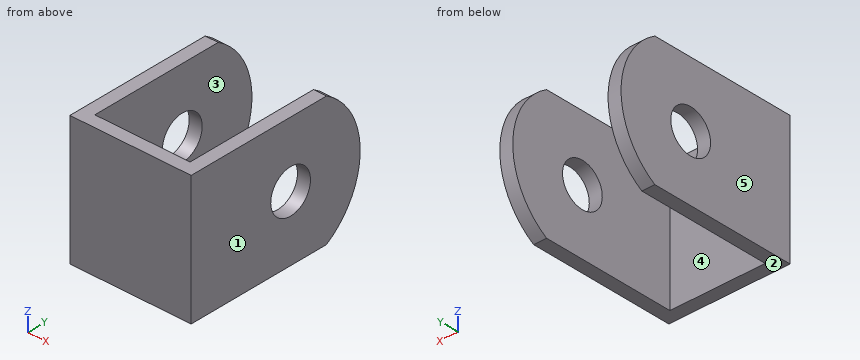
from build123d import *

# Parameters (mm, degrees)
SKETCH1_W           = 22
SKETCH1_H           = 35
BOSS_EXTRUDE1_DEPTH = 3
SKETCH2_W           = 35
SKETCH2_H           = 3
BOSS_EXTRUDE6_DEPTH = 3
BOSS_EXTRUDE7_START = 3
SKETCH4_W           = 35
SKETCH4_H           = 3
BOSS_EXTRUDE7_DEPTH = 3
SKETCH5_W           = 28
SKETCH5_H           = 2.5
CUT_EXTRUDE1_DEPTH  = 50


with BuildPart() as part:
    # Sketch1 → Boss-Extrude1 (new body)
    with BuildSketch(Plane(origin=(0, 0, 0), x_dir=(1, 0, 0), z_dir=(0, 1, 0))):
        with Locations((-45.186046512, -0.081395349)):
            Rectangle(SKETCH1_W, SKETCH1_H)
    extrude(amount=BOSS_EXTRUDE1_DEPTH)

    # Sketch2 → Boss-Extrude6 (add)
    with BuildSketch(Plane(origin=(-34.186046512, 0, 0), x_dir=(0, 0, -1), z_dir=(1, 0, 0))):
        with BuildLine():
            ThreePointArc((17.418604651, 25), (-0.081395349, 42.5), (-17.581395349, 25))
            Line((-17.581395349, 25), (-5.081395349, 25))
            ThreePointArc((-5.081395349, 25), (-0.081395349, 30), (4.918604651, 25))
            Line((4.918604651, 25), (17.418604651, 25))
        make_face()
        with BuildLine():
            Line((-5.081395349, 25), (-17.581395349, 25))
            ThreePointArc((-17.581395349, 25), (-0.081395349, 7.5), (17.418604651, 25))
            Line((17.418604651, 25), (4.918604651, 25))
            ThreePointArc((4.918604651, 25), (-0.081395349, 20), (-5.081395349, 25))
        make_face()
        with BuildLine():
            Line((-17.581395349, 25), (-17.581395349, 3))
            Line((-17.581395349, 3), (17.418604651, 3))
            Line((17.418604651, 3), (17.418604651, 25))
            ThreePointArc((17.418604651, 25), (-0.081395349, 7.5), (-17.581395349, 25))
        make_face()
        with Locations((-0.081395349, 1.5)):
            Rectangle(SKETCH2_W, SKETCH2_H)
    extrude(amount=BOSS_EXTRUDE6_DEPTH)

    # Sketch4 → Boss-Extrude7 (add)
    with BuildSketch(Plane.ZY.offset(56.186046512).offset(BOSS_EXTRUDE7_START)):
        with BuildLine():
            ThreePointArc((17.581395349, 25), (0.081395349, 42.5), (-17.418604651, 25))
            Line((-17.418604651, 25), (-4.918604651, 25))
            ThreePointArc((-4.918604651, 25), (0.081395349, 30), (5.081395349, 25))
            Line((5.081395349, 25), (17.581395349, 25))
        make_face()
        with BuildLine():
            Line((-4.918604651, 25), (-17.418604651, 25))
            ThreePointArc((-17.418604651, 25), (0.081395349, 7.5), (17.581395349, 25))
            Line((17.581395349, 25), (5.081395349, 25))
            ThreePointArc((5.081395349, 25), (0.081395349, 20), (-4.918604651, 25))
        make_face()
        with BuildLine():
            Line((-17.418604651, 25), (-17.418604651, 3))
            Line((-17.418604651, 3), (17.581395349, 3))
            Line((17.581395349, 3), (17.581395349, 25))
            ThreePointArc((17.581395349, 25), (0.081395349, 7.5), (-17.418604651, 25))
        make_face()
        with Locations((0.081395349, 1.5)):
            Rectangle(SKETCH4_W, SKETCH4_H)
    extrude(amount=-BOSS_EXTRUDE7_DEPTH)

    # Sketch5 → Cut-Extrude1 (cut)
    with BuildSketch(Plane.XZ):
        with Locations((-45.186046512, 16.331395349)):
            Rectangle(SKETCH5_W, SKETCH5_H)
        with Locations((-45.186046512, -16.168604651)):
            Rectangle(SKETCH5_W, SKETCH5_H)
    extrude(amount=-CUT_EXTRUDE1_DEPTH, mode=Mode.SUBTRACT)


solid = part.part
The model under review builds one solid part; all positions refer to its coordinate system, in mm. Face numbers are marked on the shaded views. A direction names the side the tool comes from. Round coordinates to 2 decimals unless told otherwise and drop trailing zeros. Write each loop counter-clockwise with the first axis right and the second up, starting at its lowest first coordinate (ties: lowest second). Pieces come first, ordered by that corner, then holes. Notation, with made-up numbers: M 26.25,79.25 L 58.25,79.25 A32 cw 58.25,109.25 Z; hole C 66,-6 d6. An arc over 180 degrees is marked long. Use a Markdown table: item, result. Add a question column.
Q1. We need section C-C, the plane z = 1.5. State the section outline as (x, y) points, plus the area to 3 significant figures.
Q2. To check wall thickness, follow line 1 (Z direction, x = -58, y = 25); line 2 (X direction, y = 34, z = -5); line 3 (Y direction, x = -36.75, z = -6). State the ranges of each line that lie inside material, in increasing order.
Q3. We need section D-D, the plane x = -33.5. State the section outline as (y, z) points, plus the area to 3 significant figures.
Q4. We need section A-A, the plane y = 25. State the section outline as (x, z) points.
Q5. We need section B-B, the plane y = 4.5. State the section outline as (x, z) points, plus the area to 3 significant figures.
Q6. The part is to be moulded in two halves that separate along X. For the marked faces 1, 2 and 3, say which applies: pulls with the +X half, pulls with the -X half, needs draft (parallel to the pull), parting line crosses it, or undercut.
Q7. Machinability: for the marked faces 4 and 5, which of the approach directions +Z, -Z, +X, -X, +Y, -Y give a long, thin tool a straight path to every point of the face, cutting with its end or side? Answer none if there is none.
Q8. Insertion check: pin 1 (8 mm diameter, centred on y = 25, z = 0.08, fed in from -X); pin 2 (11 mm diameter, centred on x = -48.5, z = -5.5, fed in from +Y). Each pin has a flat end and moves straight along its axis. Give the tip position at first contact, or say it passes through.
Findings below:
| question | item | result |
|---|---|---|
| 1 | outline | M -59.19,0 L -31.19,0 L -31.19,20.21 L -34.19,20.21 L -34.19,3 L -56.19,3 L -56.19,20.21 L -59.19,20.21 Z; M -59.19,29.79 L -56.19,29.79 L -56.19,42.44 L -59.19,42.44 Z; M -34.19,29.79 L -31.19,29.79 L -31.19,42.44 L -34.19,42.44 Z |
| 1 | area | 263 mm² |
| 2 | line 1 | z = -14.92 to -4.92, 5.08 to 15.08 |
| 2 | line 2 | x = -59.19 to -56.19, -34.19 to -31.19 |
| 2 | line 3 | y = 0 to 3 |
| 3 | outline | M 0,-14.92 L 34.01,-14.92 A17.5 ccw 34.01,15.08 L 0,15.08 Z; hole C 25,0.08 d10 |
| 3 | area | 1,120 mm² |
| 4 | outline | M -59.19,-14.92 L -56.19,-14.92 L -56.19,-4.92 L -59.19,-4.92 Z; M -59.19,5.08 L -56.19,5.08 L -56.19,15.08 L -59.19,15.08 Z; M -34.19,-14.92 L -31.19,-14.92 L -31.19,-4.92 L -34.19,-4.92 Z; M -34.19,5.08 L -31.19,5.08 L -31.19,15.08 L -34.19,15.08 Z |
| 5 | outline | M -59.19,-14.92 L -56.19,-14.92 L -56.19,15.08 L -59.19,15.08 Z; M -34.19,-14.92 L -31.19,-14.92 L -31.19,15.08 L -34.19,15.08 Z |
| 5 | area | 180 mm² |
| 6 | face 1 | pulls with the +X half |
| 6 | face 2 | needs draft |
| 6 | face 3 | undercut |
| 7 | face 4 | +Z, -Z, +Y |
| 7 | face 5 | +Z, -Z, -X, +Y, -Y |
| 8 | pin 1 | passes through |
| 8 | pin 2 | stops at y = 3 |
